```python
from build123d import *

# Parameters (mm, degrees)
F0_W     = 108
F0_H     = 10
F0_R     = 2
F1_DEPTH = 3
F2_SIZE  = 3


with BuildPart() as f1:
    # F0 (on Top) → F1 (new body)
    with BuildSketch(Plane.XY):
        Rectangle(F0_W, F0_H)
        with Locations((-48, 0)):
            Circle(F0_R, mode=Mode.SUBTRACT)
        with Locations((-18, 0)):
            Circle(F0_R, mode=Mode.SUBTRACT)
        with Locations((14, 0)):
            Circle(F0_R, mode=Mode.SUBTRACT)
        with Locations((48, 0)):
            Circle(F0_R, mode=Mode.SUBTRACT)
    extrude(amount=F1_DEPTH)

    # F2
    f2_edges = [f1.edges().sort_by_distance(p)[0] for p in [
        (54, 5, 1.5),
    ]]
    chamfer(f2_edges, length=F2_SIZE)


solid = f1.part
```
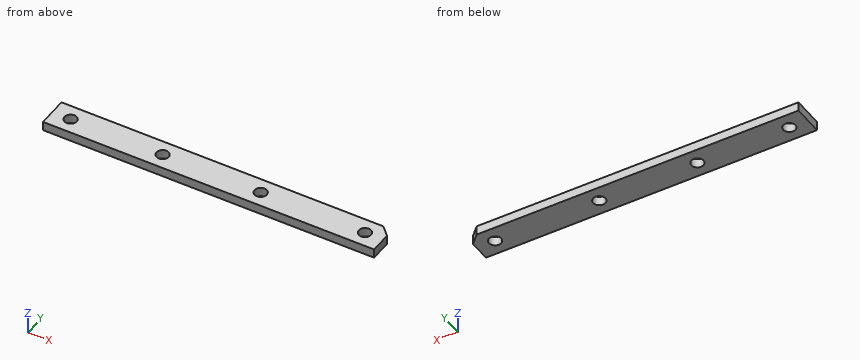
The listing builds one solid part. Answer for the finished solid, in the listing's coordinates (mm). Round coordinates to 2 decimals unless told otherwise and drop trailing zeros. Loops run counter-clockwise (first coordinate to the right, second up) from the corner with the lowest first, then second, coordinate; pieces in that order, holes last.
Q1. Given pin 1 Ø1 at (y, z) = (3, 0.5) entering from +X; pin 2 Ø3 at (x, y) = (14, 0) entering from -Z, each flat-ended and moving along its own axis, determine where each tip first touches the part or whether it passes through.
Q2. Section B-B, the plane x = 48 is taken. Determine the outline of the cut face in (y, z).
Q3. Find the intervals of material crossed by line 1 (Y direction, x = -18, z = 2.05); line 2 (X direction, y = -1.75, z = 1.4); line 3 (X direction, y = 1.25, z = 2.4), in increasing order.
Q4. Section A-A, the plane y = 0 is taken. Determine the outline of the cut face in (x, z), then the cut area to 3 significant figures.
Q5. Section D-D, the plane x = -18.5 is taken. Determine the outline of the cut face in (y, z).
Q6. Section C-C, the plane z = 1.45 is taken. Determine the outline of the cut face in (x, y).
Completed:
1. pin 1: stops at x = 53.5
1. pin 2: passes through
2. outline: (-5, 0) - (-2, 0) - (-2, 3) - (-5, 3) - close; (2, 0) - (5, 0) - (5, 3) - (2, 3) - close
3. line 1: y = -5 to -2, 2 to 5
3. line 2: x = -54 to -48.97, -47.03 to -18.97, -17.03 to 13.03, 14.97 to 47.03, 48.97 to 54
3. line 3: x = -54 to -49.56, -46.44 to -19.56, -16.44 to 12.44, 15.56 to 46.44, 49.56 to 54
4. outline: (-54, 0) - (-50, 0) - (-50, 3) - (-54, 3) - close; (-46, 0) - (-20, 0) - (-20, 3) - (-46, 3) - close; (-16, 0) - (12, 0) - (12, 3) - (-16, 3) - close; (16, 0) - (46, 0) - (46, 3) - (16, 3) - close; (50, 0) - (54, 0) - (54, 3) - (50, 3) - close
4. area: 276 mm2
5. outline: (-5, 0) - (-1.94, 0) - (-1.94, 3) - (-5, 3) - close; (1.94, 0) - (5, 0) - (5, 3) - (1.94, 3) - close
6. outline: (-54, -5) - (54, -5) - (54, 2) - (51, 5) - (-54, 5) - close; hole circle Ø4 at (-48, 0); hole circle Ø4 at (-18, 0); hole circle Ø4 at (14, 0); hole circle Ø4 at (48, 0)
